Source: CAD feature listing. Evaluate the final solid. Frame: model axes, mm. A direction names the side the tool comes from. Give positions to 0.01 mm unless a question says otherwise; leave off trailing zeros. Order: outer loops, then holes, each group sorted by start corner. A loop starts at its lowest first (then second) coordinate and runs counter-clockwise, first axis right, second up. Notation, with made-up numbers: (40, 6.5) - (68, 6.5) arc R23 cw to (68, 33.5) - close; hole circle Ø10 at (-39, 82.25). An arc over 180 degrees is marked (long way). Use CSV: the item, a comma, the result in double quotes.
```python
from build123d import *

# Parameters (mm, degrees)
BOSS_EXTRUDE1_DEPTH     = 8
BOSS_EXTRU_1_DEPTH      = 8
ESQUISSE3_W             = 12.203333334
ESQUISSE3_H             = 0.5
ENL_V_MAT_EXTRU_1_DEPTH = 39.016443811
SKETCH3_R               = 1.75
CUT_EXTRUDE1_DEPTH      = 38.969711345


with BuildPart() as part:
    # Sketch2 → Boss-Extrude1 (new body)
    with BuildSketch(Plane(origin=(0, 0, 0), x_dir=(1, 0, 0), z_dir=(0, 1, 0))):
        Polygon((12.5, 0), (2.5, 35), (-2.5, 35), (-12.5, 0), align=None)
    extrude(amount=BOSS_EXTRUDE1_DEPTH)

    # Esquisse2 → Boss.-Extru.1 (add)
    with BuildSketch(Plane(origin=(0, 0, 0), x_dir=(1, 0, 0), z_dir=(0, 1, 0))):
        Polygon((-8.901666667, 0), (-8.901666667, -2.6), (-12.001666667, -2.6), (-12.001666667, -4.6), (-3.001666667, -4.6), (-3.001666667, -2.6), (-6.101666667, -2.6), (-6.101666667, 0), align=None)
    boss_extru_1 = extrude(amount=BOSS_EXTRU_1_DEPTH)

    # Symétrie1: Boss.-Extru.1 across plane
    add(boss_extru_1.mirror(Plane(origin=(0, 0, 0), x_dir=(0, 0, 1), z_dir=(1, 0, 0))))

    # Esquisse3 → Enlèv. mat.-Extru.1 (cut, through all)
    with BuildSketch(Plane(origin=(0, 8, 0), x_dir=(1, 0, 0), z_dir=(0, 1, 0))):
        Polygon((-12.5, 0), (-8.901666667, 0), (-8.901666667, 0.5), (-12.357142857, 0.5), align=None)
        with Locations((0, 0.25)):
            Rectangle(ESQUISSE3_W, ESQUISSE3_H)
        Polygon((8.901666667, 0), (8.901666667, 0.5), (12.357142857, 0.5), (12.5, 0), align=None)
    extrude(amount=-ENL_V_MAT_EXTRU_1_DEPTH, mode=Mode.SUBTRACT)

    # Sketch3 → Cut-Extrude1 (cut, through all)
    with BuildSketch(Plane.XZ):
        with Locations(Location((0, -5.5, 0), (0, 0, 270))):
            Circle(SKETCH3_R)
    extrude(amount=-CUT_EXTRUDE1_DEPTH, mode=Mode.SUBTRACT)


solid = part.part
```
Item 1: Set-up query: faces 4 (the flat face through (3.002, 4, 4)), 5 (the flat face through (8.902, 4, 1)), 6 (the flat face through (0, 4, -0.5)). Return all of +Z, -Z, +X, -X, +Y, -Y with unobstructed straight access to the full face (end or side cutting, diameter ignored); none if empty.
Filled in:
face 4,"+Z, +Y, -Y"
face 5,"+X, +Y, -Y"
face 6,"+Y, -Y"
Item 2: Section C-C on z = -5.5. Return the cut outline in (x, y), then the cut area to 3 significant figures.
Filled in:
outline,"(-10.93, 0) - (-1.75, 0) - (-1.75, 8) - (-10.93, 8) - close; (1.75, 0) - (10.93, 0) - (10.93, 8) - (1.75, 8) - close"
area,"147 mm2"
Item 3: Section A-A on x = 0. Return the cut outline in (y, z).
Filled in:
outline,"(0, -35) - (8, -35) - (8, -7.25) - (0, -7.25) - close; (0, -3.75) - (8, -3.75) - (8, -0.5) - (0, -0.5) - close"
Item 4: First-contact query: pin 1 (1.6 mm diameter, centred on y = 5.5, z = 0.5, fed in from -X); pin 2 (1.6 mm diameter, centred on y = 6, z = 2, fed in from +X); pin 3 (3.5 mm diameter, centred on x = -4, y = 3, fed in from -Z); pin 4 (1 mm diameter, centred on y = 5.5, z = 3.5, fed in from -X). Flat tips, straight axial feed; report the tip coordinate or a pass-through.
Filled in:
pin 1,"stops at x = -8.9"
pin 2,"stops at x = 12"
pin 3,"stops at z = -35"
pin 4,"stops at x = -12"
Item 5: Section D-D on z = -24.5. Return the cut outline in (x, y).
Filled in:
outline,"(-5.5, 0) - (5.5, 0) - (5.5, 8) - (-5.5, 8) - close"
Item 6: Mould query, pull axis X, two halves, no side actions, for faces 1 (the flat face through (-8, 4, 4.6)), 2 (the flat face through (12.002, 4, 4)), 3 (the cylindrical face through (0.08, 3.94, -3.75)). Classes: released by +X, released by -X, zero draft, split by the parting line, or undercut.
Filled in:
face 1,"zero draft"
face 2,"released by +X"
face 3,"undercut"
Item 7: Section B-B on y = 4. Return the cut outline in (x, z), then the cut area to 3 significant figures.
Filled in:
outline,"(-12.36, -0.5) - (-2.5, -35) - (2.5, -35) - (12.36, -0.5) - (8.9, -0.5) - (8.9, 2.6) - (12, 2.6) - (12, 4.6) - (3, 4.6) - (3, 2.6) - (6.1, 2.6) - (6.1, -0.5) - (-6.1, -0.5) - (-6.1, 2.6) - (-3, 2.6) - (-3, 4.6) - (-12, 4.6) - (-12, 2.6) - (-8.9, 2.6) - (-8.9, -0.5) - close; hole circle Ø3.5 at (0, -5.5)"
area,"556 mm2"
Item 8: Material intervals for line 1 (X direction, y = 7.75, z = 3); line 2 (X direction, y = 4, z = -5.5); line 3 (Z direction, x = -0.75, y = 3.75), sorted ascending. Write a range as from..to.
Filled in:
line 1,"x = -12..-3, 3..12"
line 2,"x = -10.93..-1.75, 1.75..10.93"
line 3,"z = -35..-7.08, -3.92..-0.5"
